Here's how the part is built. I have some questions about the finished solid (model axes, mm). Round coordinates to 2 decimals unless told otherwise and drop trailing zeros. Order: outer loops, then holes, each group sorted by start corner. A loop starts at its lowest first (then second) coordinate and runs counter-clockwise, first axis right, second up.
```python
from build123d import *

# Parameters (mm, degrees)
SKETCH1_W                   = 3.8
SKETCH1_H                   = 15
BOSS_EXTRUDE1_DEPTH         = 2
FILLET1_RADIUS              = 1.9
FILLET1_LENGTH              = 15
FILLET1_OF_MIRROR1_2_RADIUS = 1.9
FILLET1_OF_MIRROR1_2_LENGTH = 15
SKETCH3_R                   = 1.5
CUT_EXTRUDE1_DEPTH          = 15


with BuildPart() as part:
    # Sketch1 → Boss-Extrude1 (new body)
    with BuildSketch(Plane(origin=(0, 0, 0), x_dir=(0, 0, -1), z_dir=(1, 0, 0))):
        with Locations((1.9, 7.5)):
            Rectangle(SKETCH1_W, SKETCH1_H)
    boss_extrude1 = extrude(amount=BOSS_EXTRUDE1_DEPTH)

    # Fillet1: full round fillet: the end face becomes a half cylinder, R = half its width
    fillet1_face = Plane((2, 7.5, -1.9), x_dir=(0, 1, 0), z_dir=(1, 0, 0))  # on the end face: x along it, z out of the body
    fillet1_slab = fillet1_face.offset(-FILLET1_RADIUS / 2) * Box(FILLET1_LENGTH, 2 * FILLET1_RADIUS, FILLET1_RADIUS, mode=Mode.PRIVATE)  # the body's end, R deep
    fillet1_round = Plane((0.1, 7.5, -1.9), x_dir=(1, 0, 0), z_dir=(0, 1, 0)) * Cylinder(FILLET1_RADIUS, FILLET1_LENGTH, mode=Mode.PRIVATE)  # its axis R under the face
    add(fillet1_slab - fillet1_round, mode=Mode.SUBTRACT)

    # Mirror1: Boss-Extrude1 across plane
    add(boss_extrude1.mirror(Plane.ZY))

    # Fillet1 of Mirror1 2: full round fillet: the end face becomes a half cylinder, R = half its width
    fillet1_of_mirror1_2_face = Plane((-2, 7.5, -1.9), x_dir=(0, 1, 0), z_dir=(-1, 0, 0))  # on the end face: x along it, z out of the body
    fillet1_of_mirror1_2_slab = fillet1_of_mirror1_2_face.offset(-FILLET1_OF_MIRROR1_2_RADIUS / 2) * Box(FILLET1_OF_MIRROR1_2_LENGTH, 2 * FILLET1_OF_MIRROR1_2_RADIUS, FILLET1_OF_MIRROR1_2_RADIUS, mode=Mode.PRIVATE)  # the body's end, R deep
    fillet1_of_mirror1_2_round = Plane((-0.1, 7.5, -1.9), x_dir=(-1, 0, 0), z_dir=(0, 1, 0)) * Cylinder(FILLET1_OF_MIRROR1_2_RADIUS, FILLET1_OF_MIRROR1_2_LENGTH, mode=Mode.PRIVATE)  # its axis R under the face
    add(fillet1_of_mirror1_2_slab - fillet1_of_mirror1_2_round, mode=Mode.SUBTRACT)

    # Sketch3 → Cut-Extrude1 (cut)
    with BuildSketch(Plane.XZ):
        with Locations(Location((0, -1.811318553, 0), (0, 0, 270))):
            Circle(SKETCH3_R)
    extrude(amount=-CUT_EXTRUDE1_DEPTH, mode=Mode.SUBTRACT)


solid = part.part
```
1) If we section it at C-C (y = 4): Write out the boundary of the cut face in (x, z).
2) I'm going to push flat-ended pins straight in: pin 1 (1 mm diameter, centred on x = -1, z = -3, fed in from -Y); pin 2 (1 mm diameter, centred on y = 2, z = -1, fed in from -X). Where does each tip first touch, or does it pass through?
3) We'd pull the mould along Z, two halves only. Please class faces 1 (the cylindrical face through (0.451, 7.395, -3.242)), 2 (the cylindrical face through (-2, 7.6, -1.9)): +Z half, -Z half, draft (parallel to the pull), parting line (faces both ways), or undercut.
4) If we section it at B-B (x = -0.9): Write out the boundary of the cut face in (y, z), plus the area to 3 significant figures.
5) If we section it at D-D (x = -1.7): Write out the boundary of the cut face in (y, z).
6) If we section it at A-A (z = -1.9): Write out the boundary of the cut face in (x, y), plus the area to 3 significant figures.
7) I need wall thicknesses on line 1 (X direction, y = 3.5, z = -1.35); line 2 (X direction, y = 5.25, z = -2.3); line 3 (Z direction, x = 0.85, y = 3). Which ranges of each line are inside material? Lowest first, please.
Solutions:
1. outline: (-0.1, -3.8) - (0.1, -3.8) arc R1.9 ccw to (0.1, 0) - (-0.1, 0) arc R1.9 ccw to start; hole circle Ø3 at (0, -1.81)
2. pin 1: stops at y = 0
2. pin 2: stops at x = -1.96
3. face 1: undercut
3. face 2: parting line
4. outline: (0, -3.62) - (15, -3.62) - (15, -3.01) - (0, -3.01) - close; (0, -0.61) - (15, -0.61) - (15, -0.18) - (0, -0.18) - close
4. area: 15.7 mm2
5. outline: (0, -2.92) - (15, -2.92) - (15, -0.88) - (0, -0.88) - close
6. outline: (-2, 0) - (-1.5, 0) - (-1.5, 15) - (-2, 15) - close; (1.5, 0) - (2, 0) - (2, 15) - (1.5, 15) - close
6. area: 15.1 mm2
7. line 1: x = -1.92 to -1.43, 1.43 to 1.92
7. line 2: x = -1.96 to -1.42, 1.42 to 1.96
7. line 3: z = -3.65 to -3.05, -0.58 to -0.15
